```python
from build123d import *

# Parameters (mm, degrees)
SKETCH033_W  = 8
SKETCH033_H  = 8.8
PAD011_DEPTH = 1
PAD012_DEPTH = 2
FILLET017_R  = 1


with BuildPart() as part:
    # Sketch033 → Pad011 (new body)
    with BuildSketch(Plane.XY):
        Rectangle(SKETCH033_W, SKETCH033_H)
    extrude(amount=PAD011_DEPTH)

    # Sketch034 (on Face5 of Pad011) → Pad012 (join)
    with BuildSketch(Plane(origin=(0, 0, 0), x_dir=(1, 0, 0), z_dir=(0, 0, -1))):
        with BuildLine():
            ThreePointArc((1.9, 0.6), (0, 2.5), (-1.9, 0.6))
            Line((-1.9, 0.6), (-1.9, -4.4))
            Line((-1.9, -4.4), (1.9, -4.4))
            Line((1.9, 0.6), (1.9, -4.4))
        make_face()
    extrude(amount=PAD012_DEPTH)

    # Fillet017
    fillet017_edges = [part.edges().sort_by_distance(p)[0] for p in [
        (1.9, 1.9, -2),
        (0, -2.5, -2),
        (-1.9, 1.9, -2),
        (0, 4.4, -2),
    ]]
    fillet(fillet017_edges, radius=FILLET017_R)


solid = part.part
```
Here's how the part is built. I have some questions about the finished solid (model axes, mm). A direction names the side the tool comes from. Round coordinates to 2 decimals unless told otherwise and drop trailing zeros. Order: outer loops, then holes, each group sorted by start corner. A loop starts at its lowest first (then second) coordinate and runs counter-clockwise, first axis right, second up. Notation, with made-up numbers: M 58,-35.75 L 99,-35.75 A17 cw 99,-26.75 Z; hole C 9,37.5 d5. An arc over 180 degrees is marked long. Answer as CSV lines item,"result".
Item 1: Imagine slicing it at B-B on y = -3. List the corners of the cut face in (x, z) for me, and give its area (3 significant figures).
From the geometry:
outline,"M -4,0 L 4,0 L 4,1 L -4,1 Z"
area,"8.00 mm2"
Item 2: We'd pull the mould along Y, two halves only. Please class faces 1 (the cylindrical face through (0, -2.5, -0.5)), 2 (the flat face through (4, -0.1, 0.5)), 3 (the cylindrical face through (0, 4.2, -1.6)): +Y half, -Y half, draft (parallel to the pull), parting line (faces both ways), or undercut.
From the geometry:
face 1,"-Y half"
face 2,"draft"
face 3,"+Y half"
Item 3: For pin 1 (0.5 mm diameter, centred on y = 2, z = -0.5, fed in from -X), with a flat end and sliding along its axis, tell me the tip position at first contact or that it passes through.
From the geometry:
pin 1,"x = -1.9"
Item 4: Imagine slicing it at A-A on x = -3.5. List the corners of the cut face in (y, z) for me, and give its area (3 significant figures).
From the geometry:
outline,"M -4.4,0 L 4.4,0 L 4.4,1 L -4.4,1 Z"
area,"8.80 mm2"
Item 5: Which directions (+Z, -Z, +X, -X, +Y, -Y) give clear straight access to the entire face, cutting with the end or side of a thin tool? Please do faces 4 (the flat face through (1.9, 1.9, -0.5)), 5 (the flat face through (-1.9, 1.9, -0.5)), 6 (the flat face through (-4, -0.1, 0.5)), 7 (the flat face through (-2, -2, 0)), 8 (the flat face through (0, 1, -2)).
From the geometry:
face 4,"-Z, +X, +Y, -Y"
face 5,"-Z, -X, +Y, -Y"
face 6,"+Z, -Z, -X, +Y, -Y"
face 7,"-Z, -Y"
face 8,"-Z, +X, -X, +Y, -Y"
Item 6: Please list where these lines run through material, in increasing order: L1, parallel to X at y = 2.5, z = -0.55; L2, parallel to Z at x = 1.25, y = -3.25; L3, parallel to Y at x = 0.75, z = -1.8. Write a range as [from, to].
From the geometry:
L1,"[-1.9, 1.9]"
L2,"[0, 1]"
L3,"[-1.9, 4]"
